Geometry: final body of the model. Coordinates: model frame, mm. Face numbers are marked on the shaded views. A direction names the side the tool comes from. Give positions to 0.01 mm unless a question says otherwise; leave off trailing zeros. Order: outer loops, then holes, each group sorted by start corner. A loop starts at its lowest first (then second) coordinate and runs counter-clockwise, first axis right, second up. Notation, with made-up numbers: (82, -9) - (128, -9) arc R15 cw to (128, -5) - close; hole circle Ø2 at (-36.75, 71.25). An arc over 180 degrees is marked (long way). One line per question, with ' | ' between items. Start each with the question number.
from build123d import *

# Parameters (mm, degrees)
SKETCH1_W           = 9
SKETCH1_H           = 8.2
BOSS_EXTRUDE1_DEPTH = 2.5
CHAMFER1_SIZE       = 1
SKETCH2_W           = 5
SKETCH2_H           = 0.5
CUT_EXTRUDE1_DEPTH  = 5
SKETCH3_R           = 1
CUT_EXTRUDE2_DEPTH  = 2
SKETCH4_R           = 0.15
BOSS_EXTRUDE2_DEPTH = 5
SKETCH5_R           = 0.15
BOSS_EXTRUDE3_DEPTH = 7


with BuildPart() as part:
    # Sketch1 → Boss-Extrude1 (new body, symmetric)
    with BuildSketch(Plane.XY):
        Rectangle(SKETCH1_W, SKETCH1_H)
    extrude(amount=BOSS_EXTRUDE1_DEPTH, both=True)

    # Chamfer1
    chamfer1_edges = [part.edges().sort_by_distance(p)[0] for p in [
        (4.5, 4.1, 0),
    ]]
    chamfer(chamfer1_edges, length=CHAMFER1_SIZE)

    # Sketch2 → Cut-Extrude1 (cut)
    with BuildSketch(Plane(origin=(0, 4.1, 0), x_dir=(1, 0, 0), z_dir=(0, 1, 0))):
        with Locations((0, -2.25)):
            Rectangle(SKETCH2_W, SKETCH2_H)
        with Locations((0, 2.25)):
            Rectangle(SKETCH2_W, SKETCH2_H)
    extrude(amount=-CUT_EXTRUDE1_DEPTH, mode=Mode.SUBTRACT)

    # Sketch3 → Cut-Extrude2 (cut)
    with BuildSketch(Plane(origin=(0, 4.1, 0), x_dir=(1, 0, 0), z_dir=(0, 1, 0))):
        with Locations((1.5, 0)):
            Circle(SKETCH3_R)
        with Locations((-1.5, 0)):
            Circle(SKETCH3_R)
    extrude(amount=-CUT_EXTRUDE2_DEPTH, mode=Mode.SUBTRACT)

    # Sketch4 → Boss-Extrude2 (add)
    with BuildSketch(Plane.XZ.offset(4.1)):
        with Locations((1.25, 0)):
            Circle(SKETCH4_R)
        with Locations((-3.75, 0)):
            Circle(SKETCH4_R)
    extrude(amount=BOSS_EXTRUDE2_DEPTH)

    # Sketch5 → Boss-Extrude3 (add)
    with BuildSketch(Plane.XZ.offset(4.1)):
        with Locations((-1.25, 0)):
            Circle(SKETCH5_R)
        with Locations((3.75, 0)):
            Circle(SKETCH5_R)
    extrude(amount=BOSS_EXTRUDE3_DEPTH)


solid = part.part
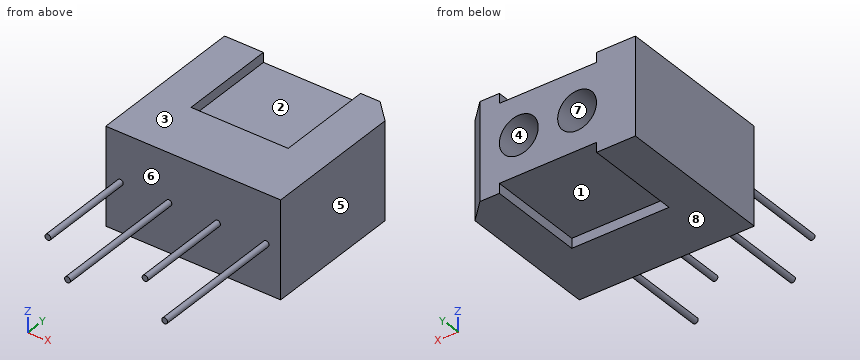
(1) Cut plane C-C, the plane y = -0.25. Return the cut outline in (x, z), plus the area to 3 significant figures.
(2) Cut plane A-A, the plane z = 0.6. Return the cut outline in (x, y), plus the area to 3 significant figures.
(3) Contact query for flat-ended pins moving along their axis: P1, Ø2, axis at x = 2, z = 0, coming from the +Y side; P2, Ø1.8, axis at x = 1.5, z = 0, coming from the +Y side; P3, Ø2.5, axis at x = 1, y = 0.5, coming from the -Z side; P4, Ø5, axis at x = -1.5, y = -8.5, coming from the -Z side. Output: stop coordinate, or through.
(4) Material intervals for line 1 along X through (y, z) = (2.8, 0); line 2 along Z through (x, y) = (1.5, 2.95); line 3 along X through (y, z) = (3.15, 0), sorted ascending. Write a range as from..to.
(5) Cut plane D-D, the plane y = -5. Return the cut outline in (x, z).
(6) Pull-direction query (Z, two-part tool) for the marked faces 6, 7 and 8; classes: +Z half, -Z half, draft (parallel to the pull), parting line (faces both ways), or undercut.
(7) Cut plane B-B, the plane x = 3.75. Return the cut outline in (y, z).
(8) Access query for the marked faces 1, 2, 3, 4 and 5. Directions: +Z, -Z, +X, -X, +Y, -Y. A direction counts if a zero-diameter tool reaches every point of the face in a straight line with its end or side. Return the directions, or none.
Results are:
1) outline: (-4.5, -2.5) - (-2.5, -2.5) - (-2.5, -2) - (2.5, -2) - (2.5, -2.5) - (4.5, -2.5) - (4.5, 2.5) - (2.5, 2.5) - (2.5, 2) - (-2.5, 2) - (-2.5, 2.5) - (-4.5, 2.5) - close | area: 40.0 mm2
2) outline: (-4.5, -4.1) - (4.5, -4.1) - (4.5, 3.1) - (3.5, 4.1) - (2.3, 4.1) - (2.3, 2.1) - (0.7, 2.1) - (0.7, 4.1) - (-0.7, 4.1) - (-0.7, 2.1) - (-2.3, 2.1) - (-2.3, 4.1) - (-4.5, 4.1) - close | area: 66.9 mm2
3) P1: y = 4.1 | P2: y = 2.1 | P3: z = -2 | P4: z = -0.15
4) line 1: -4.5..-2.5, -0.5..0.5, 2.5..4.5 | line 2: -2..-1, 1..2 | line 3: -4.5..-2.5, -0.5..0.5, 2.5..4.45
5) outline: circle Ø0.3 at (-3.75, 0); circle Ø0.3 at (-1.25, 0); circle Ø0.3 at (1.25, 0); circle Ø0.3 at (3.75, 0)
6) face 6: draft | face 7: undercut | face 8: -Z half
7) outline: (-11.1, -0.15) - (-4.1, -0.15) - (-4.1, -2.5) - (3.85, -2.5) - (3.85, 2.5) - (-4.1, 2.5) - (-4.1, 0.15) - (-11.1, 0.15) - close
8) face 1: -Z, +Y | face 2: +Z, +Y | face 3: +Z, +X, -X, +Y, -Y | face 4: +Y | face 5: +Z, -Z, +X, +Y, -Y
